Could you check a few things on this model? Use its own coordinates, in mm. Face numbers are marked on the shaded views. A direction names the side the tool comes from. Coordinates: 2 decimals unless noted, no trailing zeros. Loops run counter-clockwise (first coordinate to the right, second up) from the corner with the lowest first, then second, coordinate; pieces in that order, holes last. Notation, with made-up numbers: M -9.75,32.25 L -2.75,32.25 A10 cw -2.75,42.25 Z; hole C -18,53 d6. An arc over 180 degrees is marked long. Write each question's results on one line, items separated by ' | '.
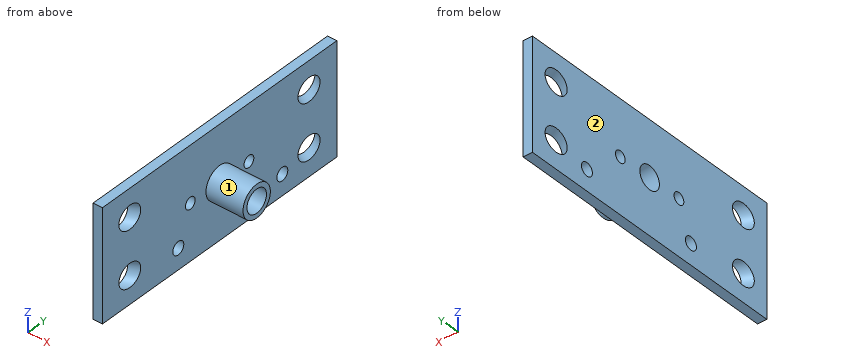
```python
from build123d import *

# Parameters (mm, degrees)
CYLINDER004_R               = 2.5
CYLINDER004_DEPTH           = 12
CYLINDER004_PITCH_ANGLE     = 90
CYLINDER003_R               = 3.5
CYLINDER003_DEPTH           = 10
CYLINDER003_PITCH_ANGLE     = 90
CYLINDER009_R               = 1.4
CYLINDER009_DEPTH           = 10
CYLINDER009_PITCH_ANGLE     = 90
CYLINDER008_R               = 1.4
CYLINDER008_DEPTH           = 10
CYLINDER008_PITCH_ANGLE     = 90
CYLINDER001_R               = 1.25
CYLINDER001_DEPTH           = 10
CYLINDER001_PITCH_ANGLE     = 90
CYLINDER002_R               = 1.25
CYLINDER002_DEPTH           = 10
CYLINDER002_PITCH_ANGLE     = 90
CYLINDER007_R               = 2.5
CYLINDER007_DEPTH           = 10
CYLINDER007_ROLL_ANGLE      = 90
CYLINDER007_PITCH_ANGLE     = 62.121453
CYLINDER007_PLACEMENT_ANGLE = 62.121453
CYLINDER006_R               = 2.5
CYLINDER006_DEPTH           = 10
CYLINDER006_ROLL_ANGLE      = 90
CYLINDER006_PITCH_ANGLE     = 62.121448
CYLINDER006_PLACEMENT_ANGLE = 62.121448
CYLINDER_R                  = 2.5
CYLINDER_DEPTH              = 10
CYLINDER_ROLL_ANGLE         = -90
CYLINDER_PITCH_ANGLE        = 63.434923
CYLINDER_PLACEMENT_ANGLE    = -63.434923
CYLINDER005_R               = 2.5
CYLINDER005_DEPTH           = 10
CYLINDER005_ROLL_ANGLE      = -90
CYLINDER005_PITCH_ANGLE     = 63.434923
CYLINDER005_PLACEMENT_ANGLE = -63.434923
BOX_W                       = 2
BOX_H                       = 60
BOX_DEPTH                   = 24


with BuildPart() as zylinder004:
    # Cylinder004 → Cylinder004 (new body)
    with BuildSketch(Plane.XY):
        Circle(CYLINDER004_R)
    extrude(amount=CYLINDER004_DEPTH)


with BuildPart() as zylinder004_1:
    # Cylinder004 pitch: moved
    add(zylinder004.part.rotate(Axis((0, 0, 0), (0, 1, 0)), CYLINDER004_PITCH_ANGLE))


with BuildPart() as zylinder004_2:
    # Cylinder004 placement: moved
    add(zylinder004_1.part.moved(Location((0, 30, 12))))


with BuildPart() as cut006:
    # Cylinder003 → Cylinder003 (new body)
    with BuildSketch(Plane.XY):
        Circle(CYLINDER003_R)
    extrude(amount=CYLINDER003_DEPTH)


with BuildPart() as cut006_1:
    # Cylinder003 pitch: moved
    add(cut006.part.rotate(Axis((0, 0, 0), (0, 1, 0)), CYLINDER003_PITCH_ANGLE))


with BuildPart() as cut006_2:
    # Cylinder003 placement: moved
    add(cut006_1.part.moved(Location((0, 30, 12))))

    # Cut006: cut Zylinder004
    add(zylinder004_2.part, mode=Mode.SUBTRACT)


with BuildPart() as zylinder009:
    # Cylinder009 → Cylinder009 (new body)
    with BuildSketch(Plane.XY):
        Circle(CYLINDER009_R)
    extrude(amount=CYLINDER009_DEPTH)


with BuildPart() as zylinder009_1:
    # Cylinder009 pitch: moved
    add(zylinder009.part.rotate(Axis((0, 0, 0), (0, 1, 0)), CYLINDER009_PITCH_ANGLE))


with BuildPart() as zylinder009_2:
    # Cylinder009 placement: moved
    add(zylinder009_1.part.moved(Location((-1, 46.05, 4.5))))


with BuildPart() as zylinder008:
    # Cylinder008 → Cylinder008 (new body)
    with BuildSketch(Plane.XY):
        Circle(CYLINDER008_R)
    extrude(amount=CYLINDER008_DEPTH)


with BuildPart() as zylinder008_1:
    # Cylinder008 pitch: moved
    add(zylinder008.part.rotate(Axis((0, 0, 0), (0, 1, 0)), CYLINDER008_PITCH_ANGLE))


with BuildPart() as zylinder008_2:
    # Cylinder008 placement: moved
    add(zylinder008_1.part.moved(Location((-1, 19.42, 4.5))))


with BuildPart() as zylinder001:
    # Cylinder001 → Cylinder001 (new body)
    with BuildSketch(Plane.XY):
        Circle(CYLINDER001_R)
    extrude(amount=CYLINDER001_DEPTH)


with BuildPart() as zylinder001_1:
    # Cylinder001 pitch: moved
    add(zylinder001.part.rotate(Axis((0, 0, 0), (0, 1, 0)), CYLINDER001_PITCH_ANGLE))


with BuildPart() as zylinder001_2:
    # Cylinder001 placement: moved
    add(zylinder001_1.part.moved(Location((0, 22.5, 12))))


with BuildPart() as zylinder002:
    # Cylinder002 → Cylinder002 (new body)
    with BuildSketch(Plane.XY):
        Circle(CYLINDER002_R)
    extrude(amount=CYLINDER002_DEPTH)


with BuildPart() as zylinder002_1:
    # Cylinder002 pitch: moved
    add(zylinder002.part.rotate(Axis((0, 0, 0), (0, 1, 0)), CYLINDER002_PITCH_ANGLE))


with BuildPart() as zylinder002_2:
    # Cylinder002 placement: moved
    add(zylinder002_1.part.moved(Location((0, 37.5, 12))))


with BuildPart() as zylinder007:
    # Cylinder007 → Cylinder007 (new body)
    with BuildSketch(Plane.XY):
        Circle(CYLINDER007_R)
    extrude(amount=CYLINDER007_DEPTH)


with BuildPart() as zylinder007_1:
    # Cylinder007 roll: moved
    add(zylinder007.part.rotate(Axis((0, 0, 0), (1, 0, 0)), CYLINDER007_ROLL_ANGLE))


with BuildPart() as zylinder007_2:
    # Cylinder007 pitch: moved
    add(zylinder007_1.part.rotate(Axis((0, 0, 0), (0, 1, 0)), CYLINDER007_PITCH_ANGLE))


with BuildPart() as zylinder007_3:
    # Cylinder007 placement: moved
    add(zylinder007_2.part.moved(Location((-2, 55, 6))).rotate(Axis((-2, 55, 6), (0, 0, 1)), CYLINDER007_PLACEMENT_ANGLE))


with BuildPart() as zylinder006:
    # Cylinder006 → Cylinder006 (new body)
    with BuildSketch(Plane.XY):
        Circle(CYLINDER006_R)
    extrude(amount=CYLINDER006_DEPTH)


with BuildPart() as zylinder006_1:
    # Cylinder006 roll: moved
    add(zylinder006.part.rotate(Axis((0, 0, 0), (1, 0, 0)), CYLINDER006_ROLL_ANGLE))


with BuildPart() as zylinder006_2:
    # Cylinder006 pitch: moved
    add(zylinder006_1.part.rotate(Axis((0, 0, 0), (0, 1, 0)), CYLINDER006_PITCH_ANGLE))


with BuildPart() as zylinder006_3:
    # Cylinder006 placement: moved
    add(zylinder006_2.part.moved(Location((-2, 55, 18))).rotate(Axis((-2, 55, 18), (0, 0, 1)), CYLINDER006_PLACEMENT_ANGLE))


with BuildPart() as zylinder:
    # Cylinder → Cylinder (new body)
    with BuildSketch(Plane.XY):
        Circle(CYLINDER_R)
    extrude(amount=CYLINDER_DEPTH)


with BuildPart() as zylinder_1:
    # Cylinder roll: moved
    add(zylinder.part.rotate(Axis((0, 0, 0), (1, 0, 0)), CYLINDER_ROLL_ANGLE))


with BuildPart() as zylinder_2:
    # Cylinder pitch: moved
    add(zylinder_1.part.rotate(Axis((0, 0, 0), (0, 1, 0)), CYLINDER_PITCH_ANGLE))


with BuildPart() as zylinder_3:
    # Cylinder placement: moved
    add(zylinder_2.part.moved(Location((-2, 5, 6))).rotate(Axis((-2, 5, 6), (0, 0, 1)), CYLINDER_PLACEMENT_ANGLE))


with BuildPart() as zylinder005:
    # Cylinder005 → Cylinder005 (new body)
    with BuildSketch(Plane.XY):
        Circle(CYLINDER005_R)
    extrude(amount=CYLINDER005_DEPTH)


with BuildPart() as zylinder005_1:
    # Cylinder005 roll: moved
    add(zylinder005.part.rotate(Axis((0, 0, 0), (1, 0, 0)), CYLINDER005_ROLL_ANGLE))


with BuildPart() as zylinder005_2:
    # Cylinder005 pitch: moved
    add(zylinder005_1.part.rotate(Axis((0, 0, 0), (0, 1, 0)), CYLINDER005_PITCH_ANGLE))


with BuildPart() as zylinder005_3:
    # Cylinder005 placement: moved
    add(zylinder005_2.part.moved(Location((-2, 5, 18))).rotate(Axis((-2, 5, 18), (0, 0, 1)), CYLINDER005_PLACEMENT_ANGLE))


with BuildPart() as fusion:
    # Box → Box (new body)
    with BuildSketch(Plane.XY):
        with Locations((1, 30)):
            Rectangle(BOX_W, BOX_H)
    extrude(amount=BOX_DEPTH)

    # Cut: cut Zylinder005
    add(zylinder005_3.part, mode=Mode.SUBTRACT)

    # Cut001: cut Zylinder
    add(zylinder_3.part, mode=Mode.SUBTRACT)

    # Cut002: cut Zylinder006
    add(zylinder006_3.part, mode=Mode.SUBTRACT)

    # Cut003: cut Zylinder007
    add(zylinder007_3.part, mode=Mode.SUBTRACT)

    # Cut004: cut Zylinder002
    add(zylinder002_2.part, mode=Mode.SUBTRACT)

    # Cut005: cut Zylinder001
    add(zylinder001_2.part, mode=Mode.SUBTRACT)

    # Cut007: cut Zylinder004
    add(zylinder004_2.part, mode=Mode.SUBTRACT)

    # Cut008: cut Zylinder008
    add(zylinder008_2.part, mode=Mode.SUBTRACT)

    # Cut009: cut Zylinder009
    add(zylinder009_2.part, mode=Mode.SUBTRACT)

    # Fusion: union Cut006
    add(cut006_2.part)


solid = fusion.part
```
(1) Will these pins go through, and if not, where does the flat tip stop? P1, Ø4, axis at x = 4.5, z = 11, coming from the +Y side; P2, Ø5, axis at y = 11.5, z = 17, coming from the +X side.
Reported:
P1: stops at y = 33.5 | P2: stops at x = 2
(2) Please list where these lines run through material, in increasing order: probe 1 along Y at (x, z) = (1, 12); probe 2 along Z at (x, y) = (0.5, 22.5); probe 3 along Z at (x, y) = (7.5, 30). Write a range as from..to.
Reported:
probe 1: y = 0..21.25, 23.75..27.5, 32.5..36.25, 38.75..60 | probe 2: z = 0..10.75, 13.25..24 | probe 3: z = 8.5..9.5, 14.5..15.5
(3) Which directions (+Z, -Z, +X, -X, +Y, -Y) give clear straight access to the entire face, cutting with the end or side of a thin tool? Please do the marked faces 1 and 2.
Reported:
face 1: +X | face 2: +Z, -Z, -X, +Y, -Y
(4) Imagine slicing it at D-D, the plane y = 37.5. List the corners of the cut face in (x, z) for me, and give its area (3 significant figures).
Reported:
outline: M 0,0 L 2,0 L 2,10.75 L 0,10.75 Z; M 0,13.25 L 2,13.25 L 2,24 L 0,24 Z | area: 43.0 mm2
(5) Imagine slicing it at C-C, the plane z = 11.5. List the corners of the cut face in (x, y) for me, and give its area (3 significant figures).
Reported:
outline: M 0,0 L 2,0 L 2,21.35 L 0,21.35 Z; M 0,23.65 L 2,23.65 L 2,26.54 L 10,26.54 L 10,27.55 L 0,27.55 Z; M 0,32.45 L 10,32.45 L 10,33.46 L 2,33.46 L 2,36.35 L 0,36.35 Z; M 0,38.65 L 2,38.65 L 2,60 L 0,60 Z | area: 117 mm2
(6) Imagine slicing it at A-A, the plane y = 19.42. List the corners of the cut face in (x, z) for me, and give its area (3 significant figures).
Reported:
outline: M 0,0 L 2,0 L 2,3.1 L 0,3.1 Z; M 0,5.9 L 2,5.9 L 2,24 L 0,24 Z | area: 42.4 mm2
(7) Imagine slicing it at B-B, the plane z = 19.75. List the corners of the cut face in (x, y) for me, and give its area (3 significant figures).
Reported:
outline: M 0,0 L 2,0 L 2,5 L 0,4 Z; M 0,8 L 2,9 L 2,50.86 L 0,51.92 Z; M 0,55.96 L 2,54.9 L 2,60 L 0,60 Z | area: 104 mm2
